Study the drawing (mm; zero at the part's minimum x, y, z) and answer. A direction names the side the tool comes from. Give positions to 0.01 mm unless a question says otherwise; leave off trailing zeros. Write each loop counter-clockwise with the first axis right and the second up, starting at its lowest first coordinate (ties: lowest second). Pieces come first, ordered by that corner, then holes.
1) Find section B-B (x = 1057.5). Determine the outline of the cut face in (y, z).
2) Find section C-C (y = 74). Determine the outline of the cut face in (x, z).
3) Determine the mould class of the marked faces 4, 5 and 6 for opening direction X: pulls with the +X half, pulls with the -X half, needs draft (parallel to the pull), parting line crosses it, or undercut.
4) Find section D-D (y = 548.5). Determine the outline of the cut face in (x, z).
5) Straight lines are drawn through the part: probe 1 along X at (y, z) = (444, 585.5); probe 2 along Y at (x, z) = (1316, 862); probe 3 along Y at (x, z) = (433, 70). For each, find the intervals that lie inside material, in ascending order.
6) A tool of negligible diameter and unlimited length cuts with its end or side. For the marked faces 1, 2 and 3, from which of +Z, -Z, +X, -X, +Y, -Y can it reach the whole face along a straight path? Write none if from no direction.
7) Given pin 1 Ø8 at (x, y) = (1444.5, 773.5) entering from +Z; pin 2 Ø8 at (x, z) = (1758, 450) entering from +Y; pin 3 Ø3 at (x, z) = (935.5, 681.5) entering from -Y, each flat-ended and moving along its own axis, determine where each tip first touches the part or whether it passes through.
8) Find section A-A (z = 890). Determine the outline of the cut face in (x, y).
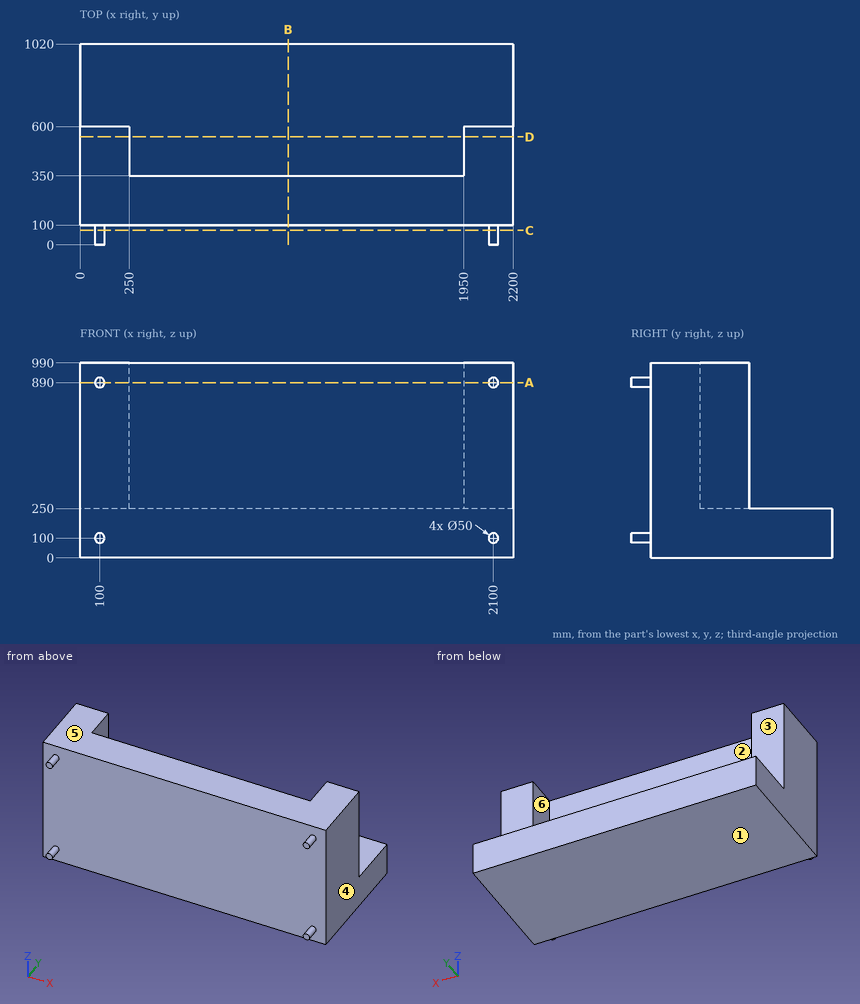
Results:
1. outline: (100, 0) - (1020, 0) - (1020, 250) - (350, 250) - (350, 990) - (100, 990) - close
2. outline: circle Ø50 at (100, 100); circle Ø50 at (100, 890); circle Ø50 at (2100, 100); circle Ø50 at (2100, 890)
3. face 4: pulls with the +X half
3. face 5: needs draft
3. face 6: undercut
4. outline: (0, 0) - (2200, 0) - (2200, 990) - (1950, 990) - (1950, 250) - (250, 250) - (250, 990) - (0, 990) - close
5. probe 1: x = 0 to 250, 1950 to 2200
5. probe 2: y = 100 to 350
5. probe 3: y = 100 to 1020
6. face 1: -Z, +X, -X, +Y, -Y
6. face 2: +Z, +Y
6. face 3: +Z, +X, -X, +Y
7. pin 1: stops at z = 250
7. pin 2: stops at y = 350
7. pin 3: stops at y = 100
8. outline: (0, 100) - (75, 100) - (75, 0) - (125, 0) - (125, 100) - (2075, 100) - (2075, 0) - (2125, 0) - (2125, 100) - (2200, 100) - (2200, 600) - (1950, 600) - (1950, 350) - (250, 350) - (250, 600) - (0, 600) - close
